The model under review builds one solid part; all positions refer to its coordinate system, in mm. A direction names the side the tool comes from. Round coordinates to 2 decimals unless told otherwise and drop trailing zeros. Write each loop counter-clockwise with the first axis right and the second up, starting at its lowest first coordinate (ties: lowest second). Pieces come first, ordered by that corner, then holes. Notation, with made-up numbers: M -14.5,-14 L 35.5,-14 A20 ccw 35.5,15 Z; hole C 18.25,59.25 d8. An arc over 180 degrees is marked long. One line per item, written item: value. Start each with the question number.
1) Take a section at A-A, the plane x = 0. Write out the cut boundary in (y, z).
2) Take a section at C-C, the plane y = 15. Write out the cut boundary in (x, z).
3) Wall thickness on probe 1 along Z at (x, y) = (-7.62, 2.8); probe 2 along X at (y, z) = (3.7, -7.65); probe 3 along Y at (x, z) = (0, 10.7): over which ranges is each line inside the solid? List them lowest first.
4) Take a section at D-D, the plane y = 23.5. Write out the cut boundary in (x, z).
5) Mouldability with a two-part tool opening along Z and no side actions: class faces 4 (the face through (-5.893, 3.849, -5.884)), 5 (the face through (-0.2, 17.3, 11.45)), 6 (the face through (8.88, 3.62, -7.82)), 7 (the face through (0, 35, 11)) as +Z half, -Z half, draft (parallel to the pull), parting line (faces both ways), or undercut.
6) Take a section at B-B, the plane z = -2.5. Write out the cut boundary in (x, y).
7) Tool access review of faces 1 (the face through (9, 5, -8)), 2 (the face through (0, 6, -11.45)), 3 (the face through (5.854, 3.849, -5.923)): name each direction out of +Z, -Z, +X, -X, +Y, -Y from which nothing blocks a thin tool from reaching the whole face with its end or side.
8) For P1, Ø2, axis at x = -7.62, z = -7.65, coming from the +Y side; P2, Ø8, axis at x = -8, y = 17.5, coming from the -Z side; P3, Ø3.5, axis at x = 7.62, z = -7.65, coming from the -Y side; P4, Ø2.5, axis at x = 7, z = -8, coming from the +Y side, all flat-tipped, find the tip position at first contact; note any pin that passes through.
from build123d import *

# Parameters (mm, degrees)
SKETCH_1_W          = 22.9
SKETCH_1_H          = 22.9
SKETCH_1_W_2        = 20.5
SKETCH_1_H_2        = 20.5
EXTRUDE_1_DEPTH     = 10
SKETCH_1_4_R        = 1.27
EXTRUDE_2_DEPTH     = 5
EXTRUDE_3_DEPTH     = 10
SKETCH_3_W          = 22.9
SKETCH_3_H          = 1.2
EXTRUDE_4_DEPTH     = 25
CUT_EXTRUDE_1_REACH = 45.365
SKETCH_4_R          = 20
SKETCH_5_R          = 2
CUT_EXTRUDE_2_DEPTH = 43.743332891


with BuildPart() as part:
    # Sketch 1 → Extrude 1 (new body)
    # profile 1 of 2: a face of its own
    with BuildSketch(Plane(origin=(0, 0, 0), x_dir=(1, 0, 0), z_dir=(0, 1, 0))):
        Rectangle(SKETCH_1_W, SKETCH_1_H)
        Rectangle(SKETCH_1_W_2, SKETCH_1_H_2, mode=Mode.SUBTRACT)
    # profile 2 of 2: a face of its own
    with BuildSketch(Plane(origin=(0, 0, 0), x_dir=(1, 0, 0), z_dir=(0, 1, 0))):
        Polygon((10.25, -10.25), (-10.25, -10.25), (-11.45, -10.25), (-11.45, -11.45), (11.45, -11.45), (11.45, -10.25), align=None)
    extrude(amount=EXTRUDE_1_DEPTH)

    # Sketch 1_4 → Extrude 2 (add)
    # profile 1 of 2: a face of its own
    with BuildSketch(Plane(origin=(0, 0, 0), x_dir=(1, 0, 0), z_dir=(0, 1, 0))):
        with BuildLine():
            Line((-5.15, 10.25), (-10.25, 10.25))
            Line((-10.25, 10.25), (-10.25, 5.18))
            Line((-10.25, 5.18), (-7.62, 5.18))
            ThreePointArc((-7.62, 5.18), (-5.87344625, 5.90344625), (-5.15, 7.65))
            Line((-5.15, 7.65), (-5.15, 10.25))
        make_face()
        with Locations(Location((-7.62, 7.65, 0), (0, 0, 270))):
            Circle(SKETCH_1_4_R, mode=Mode.SUBTRACT)
    # profile 2 of 2: a face of its own
    with BuildSketch(Plane(origin=(0, 0, 0), x_dir=(1, 0, 0), z_dir=(0, 1, 0))):
        with BuildLine():
            Line((10.25, 10.25), (5.15, 10.25))
            Line((5.15, 10.25), (5.15, 7.65))
            ThreePointArc((5.15, 7.65), (5.87344625, 5.90344625), (7.62, 5.18))
            Line((7.62, 5.18), (10.25, 5.18))
            Line((10.25, 5.18), (10.25, 10.25))
        make_face()
        with Locations(Location((7.62, 7.65, 0), (0, 0, 270))):
            Circle(SKETCH_1_4_R, mode=Mode.SUBTRACT)
    extrude(amount=EXTRUDE_2_DEPTH)

    # Sketch 1_5 → Extrude 3 (add)
    with BuildSketch(Plane(origin=(0, 0, 0), x_dir=(1, 0, 0), z_dir=(0, 1, 0))):
        Polygon((10.25, -10.25), (-10.25, -10.25), (-11.45, -10.25), (-11.45, -11.45), (11.45, -11.45), (11.45, -10.25), align=None)
    extrude(amount=EXTRUDE_3_DEPTH)

    # Sketch 3 → Extrude 4 (add)
    with BuildSketch(Plane(origin=(0, 10, 0), x_dir=(1, 0, 0), z_dir=(0, 1, 0))):
        with Locations((0, -10.85)):
            Rectangle(SKETCH_3_W, SKETCH_3_H)
    extrude(amount=EXTRUDE_4_DEPTH)

    # Sketch 4 → Cut-Extrude 1 (cut, up to next)
    with BuildSketch(Plane(origin=(0, 0, -11.45), x_dir=(-1, 0, 0), z_dir=(0, 0, -1)), mode=Mode.PRIVATE) as cut_extrude_1_sk1:
        with Locations((0, -16.398094401)):
            Circle(SKETCH_4_R)
    cut_extrude_1_tool1 = extrude(cut_extrude_1_sk1.sketch, amount=-CUT_EXTRUDE_1_REACH, mode=Mode.PRIVATE) & part.part
    add(cut_extrude_1_tool1.solids().sort_by_distance((0, -16.398094, -11.45))[0], mode=Mode.SUBTRACT)

    # Sketch 5 → Cut-Extrude 2 (cut, through all)
    with BuildSketch(Plane(origin=(0, 0, 10.25), x_dir=(-1, 0, 0), z_dir=(0, 0, -1))):
        with Locations((0, 15)):
            Circle(SKETCH_5_R)
        with Locations((0, 30)):
            Circle(SKETCH_5_R)
    extrude(amount=-CUT_EXTRUDE_2_DEPTH, mode=Mode.SUBTRACT)


solid = part.part
Checked values:
1. outline: M 3.6,-11.45 L 10,-11.45 L 10,-10.25 L 3.6,-10.25 Z; M 3.6,10.25 L 13,10.25 L 13,11.45 L 3.6,11.45 Z; M 17,10.25 L 28,10.25 L 28,11.45 L 17,11.45 Z; M 32,10.25 L 35,10.25 L 35,11.45 L 32,11.45 Z
2. outline: M -11.45,10.25 L -2,10.25 L -2,11.45 L -11.45,11.45 Z; M 2,10.25 L 11.45,10.25 L 11.45,11.45 L 2,11.45 Z
3. probe 1: z = -11.45 to -8.92, -6.38 to -5.18, 10.25 to 11.45
3. probe 2: x = -11.45 to -8.89, -6.35 to -5.15, 5.15 to 6.35, 8.89 to 11.45
3. probe 3: y = 3.6 to 13, 17 to 28, 32 to 35
4. outline: M -11.45,10.25 L 11.45,10.25 L 11.45,11.45 L -11.45,11.45 Z
5. face 4: undercut
5. face 5: +Z half
5. face 6: undercut
5. face 7: draft
6. outline: M -11.45,0 A20 cw -10.25,0.78 L -10.25,10 L -11.45,10 Z; M 10.25,0.78 A20 cw 11.45,0 L 11.45,10 L 10.25,10 Z
7. face 1: +Y
7. face 2: -Z, +X, -X, +Y, -Y
7. face 3: +Y, -Y
8. P1: passes through
8. P2: stops at z = 10.25
8. P3: stops at y = 1.27
8. P4: stops at y = 5
